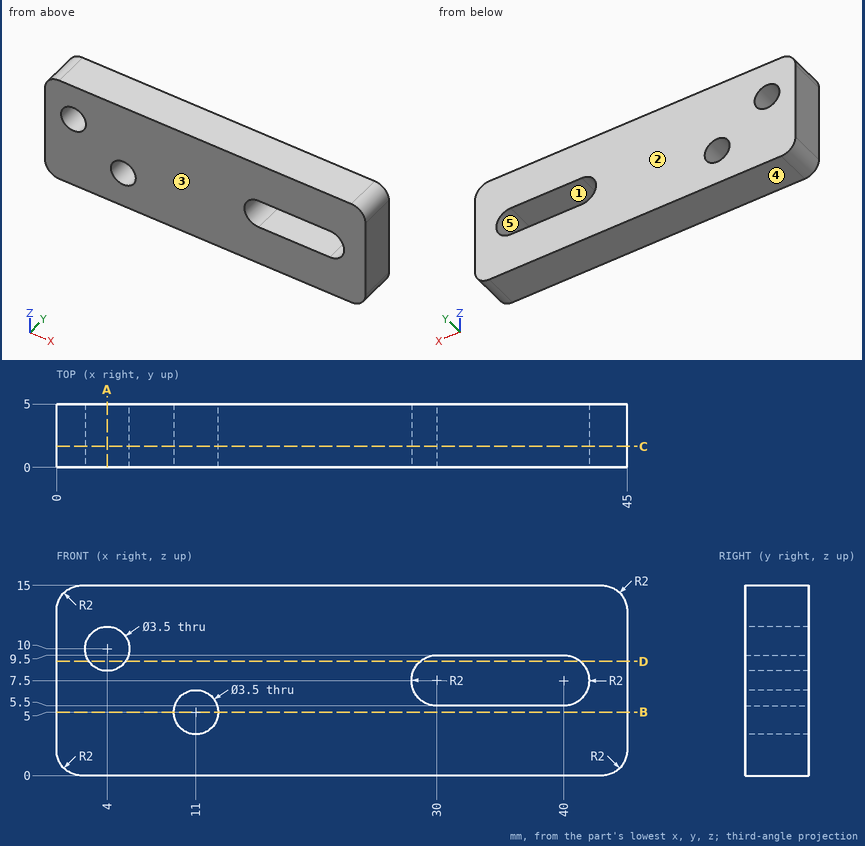
Part print with two shaded views. Sizes in mm from the minimum x, y, z corner. A direction names the side the tool comes from. Round coordinates to 2 decimals unless told otherwise and drop trailing zeros. Order: outer loops, then holes, each group sorted by start corner. A loop starts at its lowest first (then second) coordinate and runs counter-clockwise, first axis right, second up. Notation, with made-up numbers: M 7,80.5 L 54,80.5 A14 ccw 54,90.5 Z; hole C -22,25.5 d1. An arc over 180 degrees is marked long. Answer in a Markdown table with one row per item. Add a question column.
Q1. Cut at B-B on z = 5. Give the cut face in (x, y).
Q2. Cut at C-C on y = 1.65. Give the cut face in (x, z), and give its area (3 significant figures).
Q3. Cut at D-D on z = 9. Give the cut face in (x, y).
Q4. Cut at A-A on x = 4. Give the cut face in (y, z).
Q5. 3-axis set-ups, long thin cutter, end or side, ignore diameter. For the marked faces 1 and 2: which of +Z, -Z, +X, -X, +Y, -Y reach the whole face in a straight line?
Q6. Wall check: L1, parallel to X at y = 2.1, z = 10; L2, parallel to X at y = 1.6, z = 5; L3, parallel to Z at x = 4, y = 1.4. Give the ranges that are in metal, low to high. Write a range as from..to.
Q7. Mould opens along Z. For the marked faces 3, 4 and 5 say: +Z half, -Z half, draft (parallel to the pull), parting line (faces both ways), or undercut.
Established:
| question | item | result |
|---|---|---|
| 1 | outline | M 0,0 L 9.25,0 L 9.25,5 L 0,5 Z; M 12.75,0 L 45,0 L 45,5 L 12.75,5 Z |
| 2 | outline | M 0,2 A2 ccw 2,0 L 43,0 A2 ccw 45,2 L 45,13 A2 ccw 43,15 L 2,15 A2 ccw 0,13 Z; hole C 4,10 d3.5; hole C 11,5 d3.5; hole M 30,5.5 L 40,5.5 A2 ccw 40,9.5 L 30.03,9.5 A2 ccw long Z |
| 2 | area | 600 mm2 |
| 3 | outline | M 0,0 L 2.56,0 L 2.56,5 L 0,5 Z; M 5.44,0 L 28.68,0 L 28.68,5 L 5.44,5 Z; M 41.32,0 L 45,0 L 45,5 L 41.32,5 Z |
| 4 | outline | M 0,0 L 5,0 L 5,8.25 L 0,8.25 Z; M 0,11.75 L 5,11.75 L 5,15 L 0,15 Z |
| 5 | face 1 | +Y, -Y |
| 5 | face 2 | +Z, -Z, +X, -X, +Y |
| 6 | L1 | x = 0..2.25, 5.75..45 |
| 6 | L2 | x = 0..9.25, 12.75..45 |
| 6 | L3 | z = 0..8.25, 11.75..15 |
| 7 | face 3 | draft |
| 7 | face 4 | -Z half |
| 7 | face 5 | undercut |
